Check sheet for the modelled part. Datum: model origin and axes. Units: mm. A direction names the side the tool comes from. Give positions to 0.01 mm unless a question says otherwise; leave off trailing zeros. Order: outer loops, then holes, each group sorted by start corner. A loop starts at its lowest first (then second) coordinate and runs counter-clockwise, first axis right, second up.
```python
from build123d import *

# Parameters (mm, degrees)
F1_DEPTH     = 19.05
F0_W         = 26.6001702666
F0_H         = 6.2427259982
F2_DEPTH     = 6.35
F3_T1_DEPTH  = 19.05
F3_T6_DEPTH  = 31.5386260012
F3_T8_DEPTH  = 31.75
F3_T10_DEPTH = 31.75
F4_SIZE      = 0.889


# Not quite as in the source:
# - a fillet or chamfer that OpenCascade refuses, or shapes differently, is made with other operations: its cross-section is extruded or revolved along the edge and cut away or added


with BuildPart() as f1:
    # F0 (on Top) → F1 (new body)
    with BuildSketch(Plane.XY):
        with BuildLine():
            Line((7.349026072, 13.5670155287), (7.349026072, 0))
            Line((7.349026072, 0), (12.0999148667, 0))
            Line((12.0999148667, 0), (12.0999148667, 6.2427259982))
            Line((12.0999148667, 6.2427259982), (38.7000851333, 6.2427259982))
            Line((38.7000851333, 6.2427259982), (38.7000851333, 0))
            Line((38.7000851333, 0), (43.450973928, 0))
            Line((43.450973928, 0), (43.450973928, 13.5670155287))
            Line((43.450973928, 13.5670155287), (39.2939448357, 13.5670155287))
            Line((39.2939448357, 13.5670155287), (39.2939448357, 30.48))
            Line((39.2939448357, 30.48), (36.5231766516, 30.48))
            ThreePointArc((36.5231766516, 30.48), (25.4, 19.3568233484), (14.2768233484, 30.48))
            Line((14.2768233484, 30.48), (11.5060551643, 30.48))
            Line((11.5060551643, 30.48), (11.5060551643, 13.5670155287))
            Line((11.5060551643, 13.5670155287), (7.349026072, 13.5670155287))
        make_face()
    extrude(amount=F1_DEPTH)

    # F0 (on Top) → F2 (join)
    with BuildSketch(Plane.XY):
        Polygon((0, 30.48), (0, 0), (7.349026072, 0), (7.349026072, 13.5670155287), (11.5060551643, 13.5670155287), (11.5060551643, 30.48), align=None)
        with Locations((25.4, 3.1213629991)):
            Rectangle(F0_W, F0_H)
        Polygon((43.450973928, 13.5670155287), (43.450973928, 0), (50.8, 0), (50.8, 30.48), (39.2939448357, 30.48), (39.2939448357, 13.5670155287), align=None)
        with BuildLine():
            Line((7.349026072, 13.5670155287), (7.349026072, 0))
            Line((7.349026072, 0), (12.0999148667, 0))
            Line((12.0999148667, 0), (12.0999148667, 6.2427259982))
            Line((12.0999148667, 6.2427259982), (38.7000851333, 6.2427259982))
            Line((38.7000851333, 6.2427259982), (38.7000851333, 0))
            Line((38.7000851333, 0), (43.450973928, 0))
            Line((43.450973928, 0), (43.450973928, 13.5670155287))
            Line((43.450973928, 13.5670155287), (39.2939448357, 13.5670155287))
            Line((39.2939448357, 13.5670155287), (39.2939448357, 30.48))
            Line((39.2939448357, 30.48), (36.5231766516, 30.48))
            ThreePointArc((36.5231766516, 30.48), (25.4, 19.3568233484), (14.2768233484, 30.48))
            Line((14.2768233484, 30.48), (11.5060551643, 30.48))
            Line((11.5060551643, 30.48), (11.5060551643, 13.5670155287))
            Line((11.5060551643, 13.5670155287), (7.349026072, 13.5670155287))
        make_face()
    extrude(amount=-F2_DEPTH)

    # F3: fillet of radius 5.08 on 4 edges, made by hand

    # F3_s2 → F3_t1 (join)
    with BuildSketch(Plane.XY):
        with BuildLine():
            ThreePointArc((7.349026072, 13.5670155287), (10.3308658007, 15.3130269169), (11.5060551643, 18.5624659292))
            Line((11.5060551643, 18.5624659292), (11.5060551643, 13.5670155287))
            Line((11.5060551643, 13.5670155287), (7.349026072, 13.5670155287))
        make_face()
    extrude(amount=F3_T1_DEPTH)


with BuildPart() as f3_tool4:
    # F3_s5 → F3_t6 (new body)
    with BuildSketch(Plane.XY.offset(-12.4886260012)):
        with BuildLine():
            ThreePointArc((43.450973928, 13.5670155287), (40.4691341993, 15.3130269169), (39.2939448357, 18.5624659292))
            Line((39.2939448357, 18.5624659292), (39.2939448357, 13.5670155287))
            Line((39.2939448357, 13.5670155287), (43.450973928, 13.5670155287))
        make_face()
    extrude(amount=F3_T6_DEPTH)

    split(bisect_by=Plane.XY.offset(-6.35), keep=Keep.TOP)


with BuildPart() as f1_1:
    add(f1.part)

    # F3_t3: union F3_tool4
    add(f3_tool4.part)

    # F3_s9 → F3_t8 (cut)
    with BuildSketch(Plane.XY.offset(-19.05)):
        with BuildLine():
            ThreePointArc((5.08, 30.48), (1.4878975516, 28.9921024484), (0, 25.4))
            Line((0, 25.4), (0, 30.48))
            Line((0, 30.48), (5.08, 30.48))
        make_face()
    extrude(amount=F3_T8_DEPTH, mode=Mode.SUBTRACT)

    # F3_s11 → F3_t10 (cut)
    with BuildSketch(Plane.XY.offset(-19.05)):
        with BuildLine():
            ThreePointArc((45.72, 30.48), (49.3121024484, 28.9921024484), (50.8, 25.4))
            Line((50.8, 25.4), (50.8, 30.48))
            Line((50.8, 30.48), (45.72, 30.48))
        make_face()
    extrude(amount=F3_T10_DEPTH, mode=Mode.SUBTRACT)

    # F4
    f4_edges = [f1_1.edges().sort_by_distance(p)[0] for p in [
        (25.4, 19.356823, 19.05),
        (25.4, 6.242726, 19.05),
        (38.700085, 3.121363, 19.05),
        (12.099915, 3.121363, 19.05),
    ]]
    chamfer(f4_edges, length=F4_SIZE)


solid = f1_1.part
```
(1) Release check for a two-part mould opening along X. For faces 1 (the face through (26, 12, 19.05)), 2 (the face through (49.272, 29.031, -3.219)), 3 (the face through (25.648, 19.205, 18.315)), 4 (the face through (7.349, 7, 9)) record: released by +X, released by -X, zero draft, split by the parting line, or undercut.
Response values:
face 1: zero draft
face 2: released by +X
face 3: undercut
face 4: released by -X
(2) Cross-section at A-A on y = 4. Enter the section's corners in (x, z).
Response values:
outline: (0, -6.35) - (50.8, -6.35) - (50.8, 0) - (43.45, 0) - (43.45, 19.05) - (39.59, 19.05) - (38.7, 18.16) - (38.7, 0) - (12.1, 0) - (12.1, 18.16) - (11.21, 19.05) - (7.35, 19.05) - (7.35, 0) - (0, 0) - close
(3) Set-up check for faces 5 (the face through (39.294, 24, 9)), 6 (the face through (4, 15, 0)), 7 (the face through (25, 3, 0)): record each of +Z, -Z, +X, -X, +Y, -Y from which the full face is reachable in a straight line by a thin tool's end or side.
Response values:
face 5: +Z, +X, +Y
face 6: +Z, -X, +Y
face 7: +Z, -Y
(4) Cross-section at D-D on y = 8.5. Enter the section's corners in (x, z).
Response values:
outline: (0, -6.35) - (50.8, -6.35) - (50.8, 0) - (43.45, 0) - (43.45, 19.05) - (7.35, 19.05) - (7.35, 0) - (0, 0) - close
(5) Cross-section at C-C on x = 25.4. Enter the section's corners in (y, z), then the cut area to 3 significant figures.
Response values:
outline: (0, -6.35) - (19.36, -6.35) - (19.36, 18.16) - (18.47, 19.05) - (7.13, 19.05) - (6.24, 18.16) - (6.24, 0) - (0, 0) - close
area: 372 mm2
(6) Cross-section at B-B on z = 13. Enter the section's corners in (x, y), then the cut area to 3 significant figures.
Response values:
outline: (7.35, 0) - (12.1, 0) - (12.1, 6.24) - (38.7, 6.24) - (38.7, 0) - (43.45, 0) - (43.45, 13.57) arc R5.08 cw to (39.29, 18.56) - (39.29, 30.48) - (36.52, 30.48) arc R11.12 cw to (14.28, 30.48) - (11.51, 30.48) - (11.51, 18.56) arc R5.08 cw to (7.35, 13.57) - close
area: 610 mm2
(7) Material ranges on L1, parallel to X at y = 9, z = 15.5; L2, parallel to Z at x = 7.5, y = 18; L3, parallel to X at y = 4, z = 10, recorded low to high.
Response values:
L1: x = 7.35 to 43.45
L2: z = -6.35 to 0
L3: x = 7.35 to 12.1, 38.7 to 43.45
(8) Gauge pin test, flat ends, axial feed: pin 1 Ø2 at (y, z) = (5, 16) entering from -X; pin 2 Ø9 at (x, y) = (4, 20) entering from +Z; pin 3 Ø15 at (y, z) = (9, 11) entering from +X; pin 4 Ø8 at (x, z) = (5.5, 10) entering from -Y. Record the tip position at first contact, or that the pin passes through.
Response values:
pin 1: stops at x = 7.35
pin 2: stops at z = 0
pin 3: stops at x = 43.45
pin 4: stops at y = 0
